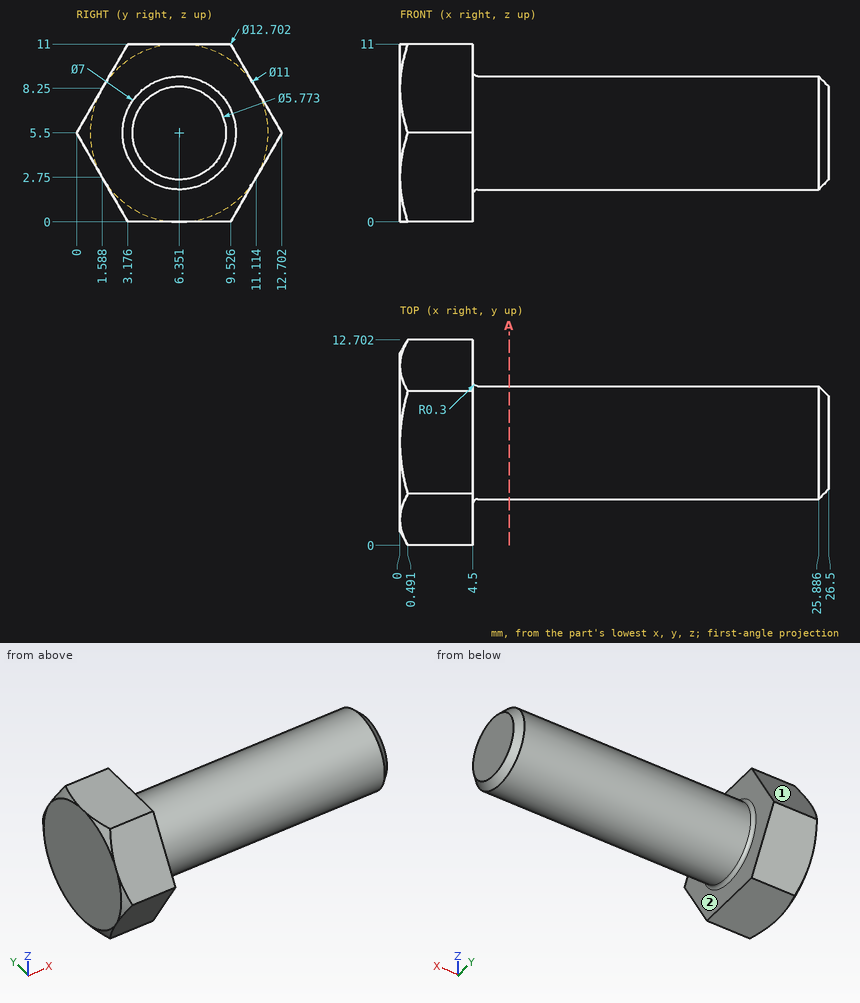
Job drawing, mm, ordinate dimensions from the low corner. One solid piece. A direction names the side the tool comes from. Coordinates: 2 decimals unless noted, no trailing zeros. Order: outer loops, then holes, each group sorted by start corner. A loop starts at its lowest first (then second) coordinate and runs counter-clockwise, first axis right, second up. Notation, with made-up numbers: (-13, 58.5) - (0, 58.5) arc R21 cw to (0, 92.5) - close; hole circle Ø7 at (11.5, -8). An arc over 180 degrees is marked (long way). Write each question's results on one line, items separated by ' | '. Start each with the question number.
Item 1: Tool access for the marked faces 1 and 2: list every direction of +Z, -Z, +X, -X, +Y, -Y with a clear straight run to the whole face (end or side of a thin tool).
Item 2: Flat gauge pins, fed straight in: pin 1 (1.5 mm diameter, centred on y = 3, z = 6.5, fed in from -X); pin 2 (2 mm diameter, centred on x = 19.5, z = 9.5, fed in from +Y) (1 decimal); pin 3 (2 mm diameter, centred on y = 2.5, z = 7.5, fed in from +X); pin 4 (2 mm diameter, centred on x = 12.5, y = 8.5, fed in from +Z) (1 decimal). Where does each tip first touch, or does it go through?
Item 3: Wall check: probe 1 along X at (y, z) = (2, 4.25); probe 2 along Z at (x, y) = (18.25, 5); probe 3 along X at (y, z) = (3.5, 4) (1 decimal). Give the ranges that are in metal, low to high. Write a range as [from, to].
Item 4: Band-saw the part on A-A on x = 6.75. Write the cut outline in (y, z), and give its area (3 significant figures).
Numbers:
1) face 1: +Z, +X, -X, +Y | face 2: +X
2) pin 1: x = 0 | pin 2: y = 8.2 | pin 3: x = 26.05 | pin 4: z = 8.8
3) probe 1: [0, 4.5] | probe 2: [2.27, 8.73] | probe 3: [0, 26.2]
4) outline: circle Ø7 at (6.35, 5.5) | area: 38.5 mm^2
